```python
from build123d import *

# Parameters (mm, degrees)
F0_R     = 1.905
F0_R_2   = 0.635
F0_R_3   = 1.524
F1_DEPTH = 3.175


with BuildPart() as f1:
    # F0 (on Front) → F1 (new body)
    with BuildSketch(Plane.XZ):
        with BuildLine():
            ThreePointArc((19.228741, 16.508046), (12.671425, 21.947552), (4.682017, 24.906601))
            ThreePointArc((4.682017, 24.906601), (0, 28.79725), (-4.682017, 24.906601))
            ThreePointArc((-4.682017, 24.906601), (-12.671425, 21.947552), (-19.228741, 16.508046))
            ThreePointArc((-19.228741, 16.508046), (-24.93915, 14.398625), (-23.910757, 8.398555))
            ThreePointArc((-23.910757, 8.398555), (-25.34285, 0), (-23.910757, -8.398555))
            ThreePointArc((-23.910757, -8.398555), (-24.93915, -14.398625), (-19.228741, -16.508046))
            ThreePointArc((-19.228741, -16.508046), (-12.671425, -21.947552), (-4.682017, -24.906601))
            ThreePointArc((-4.682017, -24.906601), (0, -28.79725), (4.682017, -24.906601))
            ThreePointArc((4.682017, -24.906601), (12.671425, -21.947552), (19.228741, -16.508046))
            ThreePointArc((19.228741, -16.508046), (24.93915, -14.398625), (23.910757, -8.398555))
            ThreePointArc((23.910757, -8.398555), (25.34285, 0), (23.910757, 8.398555))
            ThreePointArc((23.910757, 8.398555), (24.93915, 14.398625), (19.228741, 16.508046))
        make_face()
        with Locations((-20.381691, -11.767375)):
            Circle(F0_R, mode=Mode.SUBTRACT)
        with Locations((-6.6802, -11.570446)):
            Circle(F0_R_2, mode=Mode.SUBTRACT)
        with Locations((-5.1816, -8.974794)):
            Circle(F0_R_2, mode=Mode.SUBTRACT)
        with Locations((-11.570446, -6.6802)):
            Circle(F0_R_2, mode=Mode.SUBTRACT)
        with Locations((-8.974794, -5.1816)):
            Circle(F0_R_2, mode=Mode.SUBTRACT)
        with Locations((-3.683, -6.379143)):
            Circle(F0_R_2, mode=Mode.SUBTRACT)
        with Locations((-6.379143, -3.683)):
            Circle(F0_R_2, mode=Mode.SUBTRACT)
        with Locations((0, -23.53475)):
            Circle(F0_R, mode=Mode.SUBTRACT)
        with Locations((0, -13.3604)):
            Circle(F0_R_2, mode=Mode.SUBTRACT)
        with Locations((0, -10.3632)):
            Circle(F0_R_2, mode=Mode.SUBTRACT)
        with Locations((0, -7.366)):
            Circle(F0_R_2, mode=Mode.SUBTRACT)
        with Locations((5.1816, -8.974794)):
            Circle(F0_R_2, mode=Mode.SUBTRACT)
        with Locations((6.6802, -11.570446)):
            Circle(F0_R_2, mode=Mode.SUBTRACT)
        with Locations((3.683, -6.379143)):
            Circle(F0_R_2, mode=Mode.SUBTRACT)
        with Locations((6.379143, -3.683)):
            Circle(F0_R_2, mode=Mode.SUBTRACT)
        with Locations((8.974794, -5.1816)):
            Circle(F0_R_2, mode=Mode.SUBTRACT)
        with Locations((11.570446, -6.6802)):
            Circle(F0_R_2, mode=Mode.SUBTRACT)
        with Locations((20.381691, -11.767375)):
            Circle(F0_R, mode=Mode.SUBTRACT)
        with Locations((-13.3604, 0)):
            Circle(F0_R_2, mode=Mode.SUBTRACT)
        with Locations((-20.381691, 11.767375)):
            Circle(F0_R, mode=Mode.SUBTRACT)
        with Locations((-10.3632, 0)):
            Circle(F0_R_2, mode=Mode.SUBTRACT)
        with Locations((-7.366, 0)):
            Circle(F0_R_2, mode=Mode.SUBTRACT)
        with Locations((-11.570446, 6.6802)):
            Circle(F0_R_2, mode=Mode.SUBTRACT)
        with Locations((-8.974794, 5.1816)):
            Circle(F0_R_2, mode=Mode.SUBTRACT)
        with Locations((-6.379143, 3.683)):
            Circle(F0_R_2, mode=Mode.SUBTRACT)
        with Locations((-3.683, 6.379143)):
            Circle(F0_R_2, mode=Mode.SUBTRACT)
        with Locations((-6.6802, 11.570446)):
            Circle(F0_R_2, mode=Mode.SUBTRACT)
        with Locations((-5.1816, 8.974794)):
            Circle(F0_R_2, mode=Mode.SUBTRACT)
        Circle(F0_R_3, mode=Mode.SUBTRACT)
        with Locations((6.379143, 3.683)):
            Circle(F0_R_2, mode=Mode.SUBTRACT)
        with Locations((3.683, 6.379143)):
            Circle(F0_R_2, mode=Mode.SUBTRACT)
        with Locations((7.366, 0)):
            Circle(F0_R_2, mode=Mode.SUBTRACT)
        with Locations((10.3632, 0)):
            Circle(F0_R_2, mode=Mode.SUBTRACT)
        with Locations((8.974794, 5.1816)):
            Circle(F0_R_2, mode=Mode.SUBTRACT)
        with Locations((11.570446, 6.6802)):
            Circle(F0_R_2, mode=Mode.SUBTRACT)
        with Locations((0, 7.366)):
            Circle(F0_R_2, mode=Mode.SUBTRACT)
        with Locations((0, 10.3632)):
            Circle(F0_R_2, mode=Mode.SUBTRACT)
        with Locations((5.1816, 8.974794)):
            Circle(F0_R_2, mode=Mode.SUBTRACT)
        with Locations((0, 13.3604)):
            Circle(F0_R_2, mode=Mode.SUBTRACT)
        with Locations((6.6802, 11.570446)):
            Circle(F0_R_2, mode=Mode.SUBTRACT)
        with Locations((13.3604, 0)):
            Circle(F0_R_2, mode=Mode.SUBTRACT)
        with Locations((20.381691, 11.767375)):
            Circle(F0_R, mode=Mode.SUBTRACT)
        with Locations((0, 23.53475)):
            Circle(F0_R, mode=Mode.SUBTRACT)
    extrude(amount=F1_DEPTH)


solid = f1.part
```
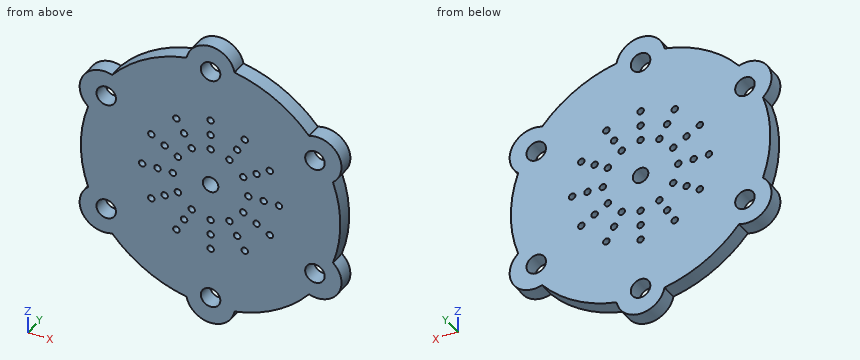
Model file for the job. Use its own axes, mm. Round coordinates to 2 decimals unless told otherwise and drop trailing zeros. Loops run counter-clockwise (first coordinate to the right, second up) from the corner with the lowest first, then second, coordinate; pieces in that order, holes last. Notation, with made-up numbers: M 22.5,68.5 L 78.5,68.5 A17 ccw 78.5,87.5 Z; hole C -37.75,33 d9. An arc over 180 degrees is marked long. Put each result on its own line as item: value. Start each with the question number.
Item 1: Cut at D-D (z = -15.5). List the corners of the cut face in (x, y) (3 decimals), then the cut area to 3 significant figures.
Item 2: Drop flat-ended pins along their axis: P1, Ø1, axis at y = -2.5, z = -22, coming from the +X side; P2, Ø1, axis at y = -2, z = -2.5, coming from the +X side. Give the stop position or say it passes through.
Item 3: Cut at A-A (z = 0). Give the number of separate pieces and of enclosed holes in the cut face, then the cut area to 3 significant figures.
Item 4: Drill centre lines: line 1 along X through (y, z) = (-2.5, -3.5); line 2 along X through (y, z) = (-0.15, -12.5); line 3 along Z through (x, y) = (22, -2.95). Where is each one in solid material? Low to high.
Answer block:
1. outline: M -24.063,-3.175 L 24.063,-3.175 L 24.063,0 L -24.063,0 Z
1. area: 153 mm2
2. P1: x = 13.42
2. P2: x = 25.26
3. separate pieces: 8
3. enclosed holes: 0
3. area: 127 mm2
4. line 1: -25.1 to -6.99, -5.77 to 5.77, 6.99 to 25.1
4. line 2: -25.55 to -22.14, -18.62 to 18.62, 22.14 to 25.55
4. line 3: -16.63 to -12.77, -10.76 to 10.76, 12.77 to 16.63
